The listing builds one solid part. Answer for the finished solid, in the listing's coordinates (mm). Face numbers are marked on the shaded views. Coordinates: 2 decimals unless noted, no trailing zeros. Order: outer loops, then holes, each group sorted by start corner. A loop starts at its lowest first (then second) coordinate and runs counter-clockwise, first axis right, second up.
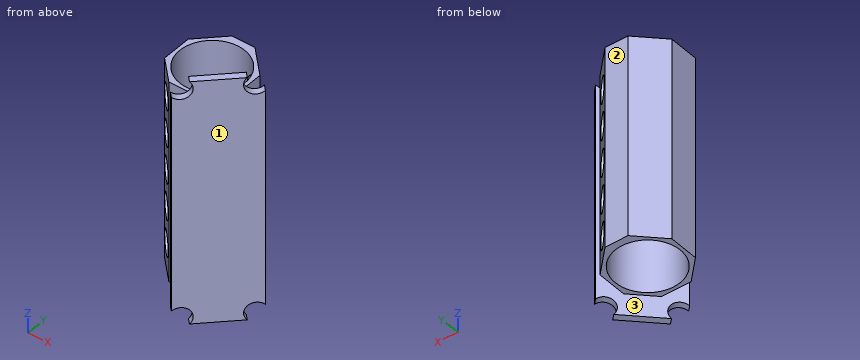
```python
from build123d import *

# Parameters (mm, degrees)
SKIZZE1_R                        = 9.65
AUFSATZ_LINEAR_AUSTRAGEN1_DEPTH  = 60
SKIZZE9_R                        = 3.5
SCHNITT_LINEAR_AUSTRAGEN8_DEPTH  = 66.276908441
SKIZZE13_W                       = 22
SKIZZE13_H                       = 72.8
AUFSATZ_LINEAR_AUSTRAGEN2_DEPTH  = 2
SKIZZE14_R                       = 3
SCHNITT_LINEAR_AUSTRAGEN12_DEPTH = 2


with BuildPart() as part:
    # Skizze1 → Aufsatz-Linear austragen1 (new body)
    with BuildSketch(Plane(origin=(0, 0, 0), x_dir=(0, 1, 0), z_dir=(0, 0, 1))):
        Polygon((11.65888225, 3.402492189), (11.65888225, -3.402492189), (4.411374439, -10.65), (-4.411374439, -10.65), (-10.65, -4.411374439), (-10.65, 4.411374439), (-4.411374439, 10.65), (4.411374439, 10.65), align=None)
        with Locations(Location((0, 0, 0), (0, 0, 270))):
            Circle(SKIZZE1_R, mode=Mode.SUBTRACT)
    extrude(amount=AUFSATZ_LINEAR_AUSTRAGEN1_DEPTH)

    # Skizze9 → Schnitt-Linear austragen8 (cut, through all)
    with BuildSketch(Plane(origin=(7.53068722, 7.53068722, 0), x_dir=(-0.7071067811865476, 0.7071067811865475, 0), z_dir=(0.7071067811865475, 0.7071067811865476, 0))):
        with Locations((0.613513233, 51.6)):
            Circle(SKIZZE9_R)
        with Locations((0.613513233, 40.6)):
            Circle(SKIZZE9_R)
        with Locations((0.613513233, 29.6)):
            Circle(SKIZZE9_R)
        with Locations((0.613513233, 18.6)):
            Circle(SKIZZE9_R)
        with Locations((0.613513233, 7.6)):
            Circle(SKIZZE9_R)
    extrude(amount=-SCHNITT_LINEAR_AUSTRAGEN8_DEPTH, mode=Mode.SUBTRACT)

    # Skizze13 → Aufsatz-Linear austragen2 (add)
    with BuildSketch(Plane(origin=(7.53068722, -7.53068722, 0), x_dir=(0.7071067811865477, 0.7071067811865475, 0), z_dir=(0.7071067811865475, -0.7071067811865477, 0))):
        with Locations((0, 30)):
            Rectangle(SKIZZE13_W, SKIZZE13_H)
    extrude(amount=AUFSATZ_LINEAR_AUSTRAGEN2_DEPTH)

    # Skizze14 → Schnitt-Linear austragen12 (cut)
    with BuildSketch(Plane(origin=(8.944900782, -8.944900782, 0), x_dir=(0.7071067811865478, 0.7071067811865474, 0), z_dir=(0.7071067811865474, -0.7071067811865478, 0))):
        with Locations((8.88, 64.28)):
            Circle(SKIZZE14_R)
        with Locations((-8.88, -4.28)):
            Circle(SKIZZE14_R)
        with Locations((8.88, -4.28)):
            Circle(SKIZZE14_R)
        with Locations((-8.88, 64.28)):
            Circle(SKIZZE14_R)
    extrude(amount=-SCHNITT_LINEAR_AUSTRAGEN12_DEPTH, mode=Mode.SUBTRACT)


solid = part.part
```
1) The mould has two halves that part along X. Classify the marked faces 1, 2 and 3: released by +X, released by -X, zero draft, split by the parting line, or undercut.
2) Each of these flat-tipped pins is pushed along its axis until it touches: P1, Ø12, axis at y = -9.5, z = 12.5, coming from the +X side; P2, Ø5, axis at x = 10.5, y = -13.5, coming from the +Z side; P3, Ø4.5, axis at x = 0, z = 26, coming from the -Y side; P4, Ø6.5, axis at x = 2.5, y = 6, coming from the -Z side. Where does it stop, or does it pass through?
3) A cutting plane is placed at C-C, the plane y = 7.75. Count the separate pieces of the cut face and the enclosed holes in it, plus the area to 3 significant figures.
4) A cutting plane is placed at B-B, the plane z = 53. Write down the section's boundary in (x, y).
5) A cutting plane is placed at A-A, the plane z = 24. Write down the section's boundary in (x, y).
6) Straight lines are drawn through the part: probe 1 along Y at (x, z) = (0, 20); probe 2 along X at (y, z) = (-2.5, 10.5); probe 3 along X at (y, z) = (-1.5, 30.5). For each, find the intervals that lie inside material, in ascending order.
Working result:
1. face 1: released by +X
1. face 2: zero draft
1. face 3: undercut
2. P1: stops at x = 14.39
2. P2: passes through
2. P3: stops at y = -16.72
2. P4: stops at z = 0
3. separate pieces: 7
3. enclosed holes: 0
3. area: 133 mm2
4. outline: (-10.65, -4.41) - (-10.23, -4.83) - (-8.97, -3.56) arc R9.65 cw to (3.56, 8.97) - (4.83, 10.23) - (3.4, 11.66) - (-3.4, 11.66) - (-10.65, 4.41) - close; (-5.7, -9.37) - (-4.41, -10.65) - (4.41, -10.65) - (-0.25, -15.31) - (1.17, -16.72) - (16.72, -1.17) - (15.31, 0.25) - (10.65, -4.41) - (10.65, 4.41) - (9.37, 5.7) - (8.41, 4.74) arc R9.65 cw to (-4.74, -8.41) - close
5. outline: (-10.65, -4.41) - (-4.41, -10.65) - (4.41, -10.65) - (-0.25, -15.31) - (1.17, -16.72) - (16.72, -1.17) - (15.31, 0.25) - (10.65, -4.41) - (10.65, 4.41) - (3.4, 11.66) - (-3.4, 11.66) - (-10.65, 4.41) - close; hole circle Ø19.3 at (0, 0)
6. probe 1: y = -15.56 to -15.06, -10.65 to -9.65, 9.65 to 11.66
6. probe 2: x = -10.65 to -9.32, 9.32 to 10.65, 12.56 to 15.39
6. probe 3: x = -10.65 to -9.53, 9.53 to 10.65, 13.56 to 16.39
